Geometry: final body of the model. Coordinates: model frame, mm. A direction names the side the tool comes from. Round coordinates to 2 decimals unless told otherwise and drop trailing zeros. Loops run counter-clockwise (first coordinate to the right, second up) from the corner with the lowest first, then second, coordinate; pieces in that order, holes last. Notation, with made-up numbers: M 77,-4.75 L 85,-4.75 A31 ccw 85,19.25 Z; hole C 67.5,-17 d10. An arc over 180 degrees is marked long. Return JSON: item names as keys, results as strings.
from build123d import *

# Parameters (mm, degrees)
SKETCH_1_W          = 200
SKETCH_1_H          = 80
EXTRUDE_1_DEPTH     = 1
CUT_EXTRUDE_1_REACH = 3
SKETCH_3_R          = 1.5
CUT_EXTRUDE_2_DEPTH = 10


with BuildPart() as part:
    # 草图1 → 凸台-拉伸1 (new body)
    with BuildSketch(Plane(origin=(0, 0, 0), x_dir=(1, 0, 0), z_dir=(0, 1, 0))):
        Rectangle(SKETCH_1_W, SKETCH_1_H)
    extrude(amount=EXTRUDE_1_DEPTH)

    # 草图2 → 切除-拉伸1 (cut, up to next)
    with BuildSketch(Plane(origin=(0, 1, 0), x_dir=(1, 0, 0), z_dir=(0, 1, 0)), mode=Mode.PRIVATE) as cut_extrude_1_sk1:
        with BuildLine():
            Line((0, 25), (70, 25))
            ThreePointArc((70, 25), (90, 5), (70, -15))
            Line((70, -15), (0, -15))
            ThreePointArc((0, -15), (-20, 5), (0, 25))
        make_face()
    cut_extrude_1_tool1 = extrude(cut_extrude_1_sk1.sketch, amount=-CUT_EXTRUDE_1_REACH, mode=Mode.PRIVATE) & part.part
    add(cut_extrude_1_tool1.solids().sort_by_distance((35, 1, -5))[0], mode=Mode.SUBTRACT)

    # 草图3 → 切除-拉伸2 (cut)
    with BuildSketch(Plane(origin=(0, 1, 0), x_dir=(1, 0, 0), z_dir=(0, 1, 0))):
        with Locations((-50, 37)):
            Circle(SKETCH_3_R)
        with Locations((50, 37)):
            Circle(SKETCH_3_R)
        with Locations((50, -37)):
            Circle(SKETCH_3_R)
        with Locations((-50, -37)):
            Circle(SKETCH_3_R)
        with Locations((-97, 0)):
            Circle(SKETCH_3_R)
        with Locations((97, 0)):
            Circle(SKETCH_3_R)
    extrude(amount=-CUT_EXTRUDE_2_DEPTH, mode=Mode.SUBTRACT)


solid = part.part
Q1. Material intervals for L1, parallel to Z at x = 50, y = 0.5; L2, parallel to Z at x = -50, y = 0.45; L3, parallel to X at y = 0.4, z = 37, sorted ascending.
Determined:
{"L1": "z = -40 to -38.5, -35.5 to -25, 15 to 35.5, 38.5 to 40", "L2": "z = -40 to -38.5, -35.5 to 35.5, 38.5 to 40", "L3": "x = -100 to -51.5, -48.5 to 48.5, 51.5 to 100"}
Q2. Section query A-A (y = 0.55). Output: boundary loops of the cut face in (x, z), plus the area to 3 significant figures.
Determined:
{"outline": "M -100,-40 L 100,-40 L 100,40 L -100,40 Z; hole C -97,0 d3; hole C -50,-37 d3; hole C -50,37 d3; hole M 0,-25 L 70,-25 A20 ccw 70,15 L 0,15 A20 ccw Z; hole C 50,-37 d3; hole C 50,37 d3; hole C 97,0 d3", "area": "11,900 mm^2"}
Q3. Pull-direction query (X, two-part tool) for faces 1 (the cylindrical face through (89.995, 0.507, -5.44)), 2 (the flat face through (-24, 1, -1)); classes: pulls with the +X half, pulls with the -X half, needs draft (parallel to the pull), parting line crosses it, or undercut.
Determined:
{"face 1": "undercut", "face 2": "needs draft"}
Q4. Reachability of faces 3 (the flat face through (-24, 0, -1)), 4 (the cylindrical face through (-19.995, 0.507, -4.56)) from +Z, -Z, +X, -X, +Y, -Y: full face, straight path, thin tool, end or side. Return the list, or none.
Determined:
{"face 3": "+Z, -Z, +X, -X, -Y", "face 4": "+Y, -Y"}
Q5. Pin query (flat end, axial travel): pin 1 (4 mm diameter, centred on x = -50, z = -37, fed in from -Y). Return the tip coordinate at first contact, or that it passes through.
Determined:
{"pin 1": "stops at y = 0"}
Q6. Section query C-C (z = -23). Output: boundary loops of the cut face in (x, y), plus the area to 3 significant figures.
Determined:
{"outline": "M -100,0 L -8.72,0 L -8.72,1 L -100,1 Z; M 78.72,0 L 100,0 L 100,1 L 78.72,1 Z", "area": "113 mm^2"}
Q7. Section query B-B (x = 58.5). Output: boundary loops of the cut face in (y, z), plus the area to 3 significant figures.
Determined:
{"outline": "M 0,-40 L 1,-40 L 1,-25 L 0,-25 Z; M 0,15 L 1,15 L 1,40 L 0,40 Z", "area": "40.0 mm^2"}
